Work out the finished part from the listing and answer in its coordinate system (mm). A direction names the side the tool comes from. Coordinates: 2 decimals unless noted, no trailing zeros. Write each loop counter-clockwise with the first axis right and the second up, starting at its lowest first coordinate (ties: lowest second). Pieces come first, ordered by that corner, then holes. Notation, with made-up numbers: (-37.75, 67) - (-10.75, 67) arc R25 ccw to (-10.75, 88) - close; hole circle Ø3 at (-38.5, -9). An arc over 180 degrees is marked (long way). Use a Markdown table: item, result. Add a question column.
(1) Given pin 1 Ø2 at (y, z) = (1, -14.5) entering from -X; pin 2 Ø1.5 at (y, z) = (2, 20) entering from +X; pin 3 Ø3 at (x, y) = (8.5, 1.5) entering from -Z; pin 4 Ø11.5 at (x, z) = (0, 0) entering from +Y, each flat-ended and moving along its own axis, determine where each tip first touches the part or whether it passes through.
(2) A tool of negligible diameter and unlimited length cuts with its end or side. For faces 1 (the face through (36.98, 3.13, -22.7)), 2 (the face through (-10.01, 5.06, -31.8)), from which of +Z, -Z, +X, -X, +Y, -Y can it reach the whole face along a straight path? Write none if from no direction.
(3) For a pull along X with two mould halves and no side action, classify faces 3 (the face through (36, 6.35, 11)), 4 (the face through (-0.94, 3.13, 50.79)), 5 (the face through (1.38, 3.13, 6.2)) as released by +X, released by -X, zero draft, split by the parting line, or undercut.
(4) The part is cut by section D-D, the plane z = -27. Give the vertices of the cut face in (x, y), then the cut area to 3 significant figures.
(5) The part is cut by section A-A, the plane y = 5.25. State how many separate pieces and enclosed holes the cut face has, then the cut area to 3 significant figures.
(6) The part is cut by section C-C, the plane x = 0. Give the vertices of the cut face in (y, z), then the cut area to 3 significant figures.
(7) Find the intervals of material crossed by line 1 (Z direction, x = -17, y = 4.75); line 2 (Z direction, x = 10.5, y = 4.5); line 3 (Y direction, x = 17, z = 30), in increasing order. Write a range as from..to.
(8) The part is cut by section B-B, the plane z = 0. Give the vertices of the cut face in (x, y), then the cut area to 3 significant figures.
from build123d import *

# Parameters (mm, degrees)
F_1_2_0_5_DIAMETER_HOLE1_D   = 12.7
F_1_1_DIAMETER_HOLE1_D       = 25.4
F_1_8_0_125_DIAMETER_HOLE1_D = 3.175


with BuildPart() as part:
    # Sketch1 → Revolve1 (revolve)
    with BuildSketch(Plane.XY, mode=Mode.PRIVATE) as revolve1_sk:
        Polygon((-33.3375, 6.35), (-33.3375, 3.81), (-36.8935, 3.81), (-36.8935, 6.35), (-50.8, 6.35), (-50.8, 0), (0, 0), (0, 6.35), align=None)
    revolve(revolve1_sk.sketch.rotate(Axis((0, 0, 0), (0, 1, 0)), 270), axis=Axis((0, 0, 0), (0, 1, 0)))

    # 1/2 (0.5) Diameter Hole1 (through all)
    with Locations(Plane(origin=(0, 6.35, 0), x_dir=(1, 0, 0), z_dir=(0, 1, 0))):
        with Locations((0, 0)):
            Hole(F_1_2_0_5_DIAMETER_HOLE1_D / 2)

    # 1 (1) Diameter Hole1 (through all)
    with Locations(Plane(origin=(0, 6.35, 0), x_dir=(1, 0, 0), z_dir=(0, 1, 0))):
        with Locations((50.8, 0), (-50.8, 0)):
            Hole(F_1_1_DIAMETER_HOLE1_D / 2)

    # 1/8 (0.125) Diameter Hole1 (through all)
    with Locations(Plane(origin=(0, 6.35, 0), x_dir=(1, 0, 0), z_dir=(0, 1, 0))):
        with Locations((38.494829198, 22.225)):
            Hole(F_1_8_0_125_DIAMETER_HOLE1_D / 2)


solid = part.part
Model answer:
| question | item | result |
|---|---|---|
| 1 | pin 1 | x = -48.97 |
| 1 | pin 2 | x = 47.01 |
| 1 | pin 3 | z = -50.32 |
| 1 | pin 4 | through |
| 2 | face 1 | +Y, -Y |
| 2 | face 2 | +Y |
| 3 | face 3 | zero draft |
| 3 | face 4 | split by the parting line |
| 3 | face 5 | undercut |
| 4 | outline | (-43.03, 0) - (43.03, 0) - (43.03, 6.35) - (25.14, 6.35) - (25.14, 3.81) - (19.55, 3.81) - (19.55, 6.35) - (-19.55, 6.35) - (-19.55, 3.81) - (-25.14, 3.81) - (-25.14, 6.35) - (-43.03, 6.35) - close |
| 4 | area | 518 mm^2 |
| 5 | separate pieces | 2 |
| 5 | enclosed holes | 3 |
| 5 | area | 6,710 mm^2 |
| 6 | outline | (0, -50.8) - (6.35, -50.8) - (6.35, -36.89) - (3.81, -36.89) - (3.81, -33.34) - (6.35, -33.34) - (6.35, -6.35) - (0, -6.35) - close; (0, 6.35) - (6.35, 6.35) - (6.35, 33.34) - (3.81, 33.34) - (3.81, 36.89) - (6.35, 36.89) - (6.35, 50.8) - (0, 50.8) - close |
| 6 | area | 546 mm^2 |
| 7 | line 1 | -47.87..-32.74, -28.68..28.68, 32.74..47.87 |
| 7 | line 2 | -49.7..-35.37, -31.64..31.64, 35.37..49.7 |
| 7 | line 3 | 0..3.81 |
| 8 | outline | (-38.1, 0) - (-6.35, 0) - (-6.35, 6.35) - (-33.34, 6.35) - (-33.34, 3.81) - (-36.89, 3.81) - (-36.89, 6.35) - (-38.1, 6.35) - close; (6.35, 0) - (38.1, 0) - (38.1, 6.35) - (36.89, 6.35) - (36.89, 3.81) - (33.34, 3.81) - (33.34, 6.35) - (6.35, 6.35) - close |
| 8 | area | 385 mm^2 |
